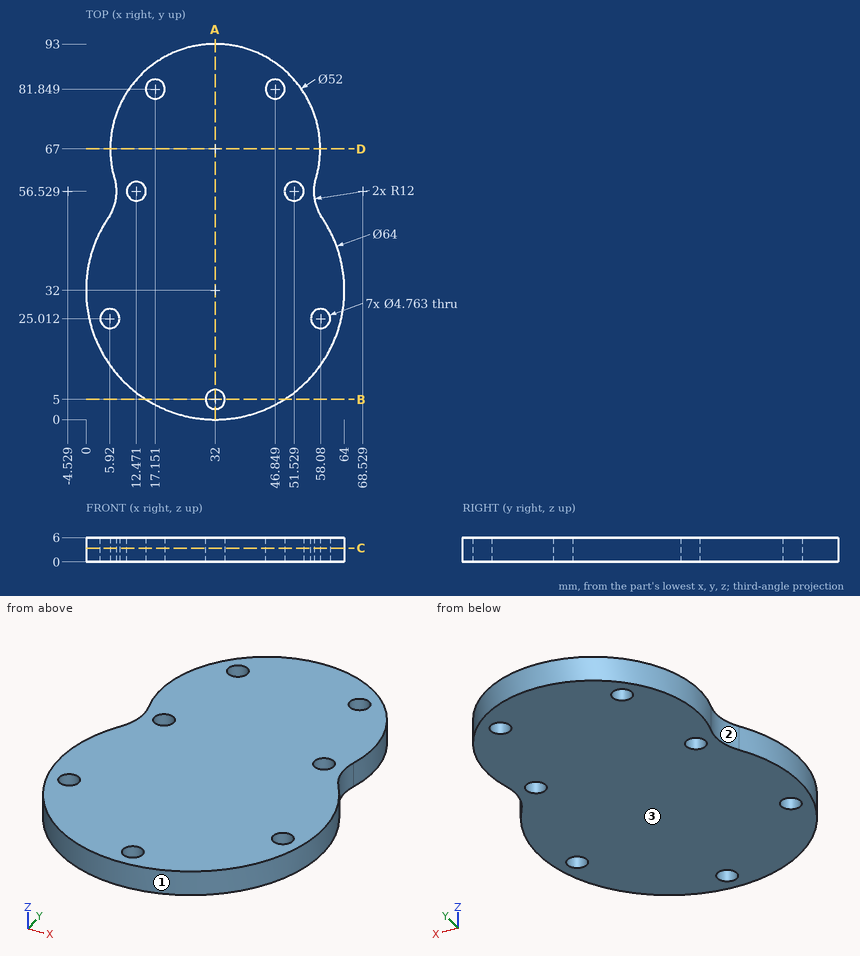
Verification items for this drawing (mm, ordinates from the low corner). Give positions to 0.01 mm unless a question says otherwise; leave off trailing zeros. Write each loop counter-clockwise with the first axis right and the second up, starting at its lowest first coordinate (ties: lowest second). Pieces come first, ordered by that corner, then holes. Notation, with made-up numbers: (-22.5, -32) -> (-18.5, -32) arc R10 cw to (-18.5, -27) -> close; hole circle Ø6 at (85.5, -17.75). An arc over 180 degrees is marked (long way). Use CSV: the item, a comma, the result in double quotes. Start each with the question number.
Q1. Cross-section at D-D on y = 67. Enter the section's corners in (x, z).
Q2. Cross-section at C-C on z = 3.4. Count the separate pieces of the cut face and the enclosed holes in it, and give its area (3 significant figures).
Q3. Cross-section at A-A on x = 32. Enter the section's corners in (y, z).
Q4. Cross-section at B-B on y = 5. Enter the section's corners in (x, z) (1 decimal).
Q5. Depth check by flat-ended pin: P1, Ø1, axis at y = 67.5, z = 1.5, coming from the +X side; P2, Ø4, axis at x = 51.53, y = 56.53, coming from the -Z side; P3, Ø3, axis at x = 47, z = 5, coming from the +Y side; P4, Ø1, axis at y = 22.5, z = 5, coming from the +X side. Enter the tip coordinate at first touch or a pass-through.
Q6. Release check for a two-part mould opening along Y. For the marked faces 1, 2 and 3 record: +Y half, -Y half, draft (parallel to the pull), parting line (faces both ways), or undercut.
Q7. Scan lines: line 1 along X through (y, z) = (82, 1.75) (1 decimal); line 2 along Y through (x, z) = (15, 4.8) (1 decimal); line 3 along X through (y, z) = (66.5, 3.75) (1 decimal). Record each from-to range of solid material in increasing order.
Working result:
1,outline,"(6, 0) -> (58, 0) -> (58, 6) -> (6, 6) -> close"
2,separate pieces,"1"
2,enclosed holes,"7"
2,area,"4,490 mm^2"
3,outline,"(0, 0) -> (2.62, 0) -> (2.62, 6) -> (0, 6) -> close; (7.38, 0) -> (93, 0) -> (93, 6) -> (7.38, 6) -> close"
4,outline,"(14.8, 0) -> (29.6, 0) -> (29.6, 6) -> (14.8, 6) -> close; (34.4, 0) -> (49.2, 0) -> (49.2, 6) -> (34.4, 6) -> close"
5,P1,"stops at x = 58"
5,P2,"passes through"
5,P3,"stops at y = 89.22"
5,P4,"stops at x = 62.71"
6,face 1,"parting line"
6,face 2,"undercut"
6,face 3,"draft"
7,line 1,"x = 10.8 to 14.8, 19.5 to 44.5, 49.2 to 53.2"
7,line 2,"y = 4.9 to 80.8, 82.9 to 86.7"
7,line 3,"x = 6 to 58"
